Can you work these out from the drawing? Everything is in mm from the part's minimum corner. Round coordinates to 2 decimals unless told otherwise and drop trailing zeros. Write each loop counter-clockwise with the first axis right and the second up, starting at its lowest first coordinate (ties: lowest second). Pieces come first, ordered by that corner, then holes. Notation, with made-up numbers: (59, 70) -> (114, 70) arc R25 cw to (114, 87) -> close; hole circle Ø7 at (23.5, 62.5). An arc over 180 degrees is marked (long way). Write item = value, one per line. Start each with the question number.
1) Imagine slicing it at D-D, the plane z = 57.15. Please give me the cut outline in (x, y).
2) Imagine slicing it at B-B, the plane x = 57.15. Please give me the cut outline in (y, z), then the cut area to 3 significant figures.
3) I'm going to push a flat-ended pin straight in: pin 1 (2 mm diameter, centred on x = 127, z = 57.15, fed in from -Y). Where does the tip first touch, or does it pass through?
4) If I drill on line 1 (Z direction, x = 127, y = 0.9); line 2 (X direction, y = 1.25, z = 12.7); line 3 (X direction, y = 2.4, z = 19.05), over which ranges is the centre line in solid material (lowest first)?
5) Imagine slicing it at C-C, the plane z = 12.7. Please give me the cut outline in (x, y), then the cut area to 3 significant figures.
6) Imagine slicing it at A-A, the plane y = 1.55. State how many separate pieces and enclosed holes the cut face has, then the cut area to 3 significant figures.
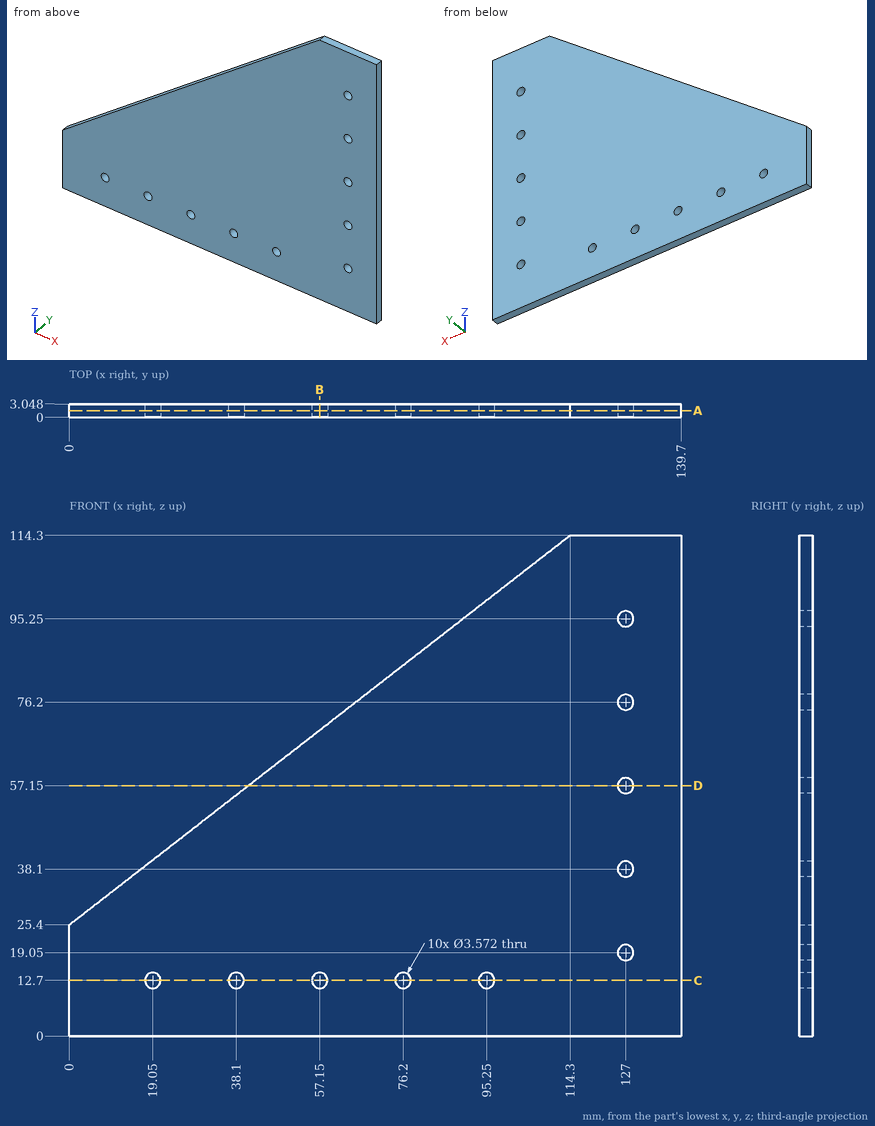
Reported:
q1.outline = (40.82, 0) -> (125.21, 0) -> (125.21, 3.05) -> (40.82, 3.05) -> close; (128.79, 0) -> (139.7, 0) -> (139.7, 3.05) -> (128.79, 3.05) -> close
q2.outline = (0, 0) -> (3.05, 0) -> (3.05, 10.91) -> (0, 10.91) -> close; (0, 14.49) -> (3.05, 14.49) -> (3.05, 69.85) -> (0, 69.85) -> close
q2.area = 202 mm²
q3.pin_1 = through
q4.line_1 = 0 to 17.26, 20.84 to 36.31, 39.89 to 55.36, 58.94 to 74.41, 77.99 to 93.46, 97.04 to 114.3
q4.line_2 = 0 to 17.26, 20.84 to 36.31, 39.89 to 55.36, 58.94 to 74.41, 77.99 to 93.46, 97.04 to 139.7
q4.line_3 = 0 to 125.21, 128.79 to 139.7
q5.outline = (0, 0) -> (17.26, 0) -> (17.26, 3.05) -> (0, 3.05) -> close; (20.84, 0) -> (36.31, 0) -> (36.31, 3.05) -> (20.84, 3.05) -> close; (39.89, 0) -> (55.36, 0) -> (55.36, 3.05) -> (39.89, 3.05) -> close; (58.94, 0) -> (74.41, 0) -> (74.41, 3.05) -> (58.94, 3.05) -> close; (77.99, 0) -> (93.46, 0) -> (93.46, 3.05) -> (77.99, 3.05) -> close; (97.04, 0) -> (139.7, 0) -> (139.7, 3.05) -> (97.04, 3.05) -> close
q5.area = 371 mm²
q6.separate_pieces = 1
q6.enclosed_holes = 10
q6.area = 10,800 mm²
